Check sheet for the modelled part. Datum: model origin and axes. Units: mm. A direction names the side the tool comes from. Round coordinates to 2 decimals unless told otherwise and drop trailing zeros. Write each loop counter-clockwise with the first axis right and the second up, starting at its lowest first coordinate (ties: lowest second). Pieces come first, ordered by that corner, then holes. Notation, with made-up numbers: (38.5, 39) -> (51.5, 39) arc R23 cw to (51.5, 65) -> close; hole circle Ø11 at (8, -35). An arc over 180 degrees is marked (long way). Answer as a JSON object with one key per item and string values. Group by question number.
```python
from build123d import *

# Parameters (mm, degrees)
SKETCH_1_W      = 12.4
SKETCH_1_H      = 5
SKETCH_1_R      = 1.25
SKETCH_1_W_2    = 5
SKETCH_1_H_2    = 11.3
EXTRUDE_1_DEPTH = 3
SKETCH_2_W      = 3
SKETCH_2_H      = 16.3
EXTRUDE_2_DEPTH = 12
EXTRUDE_3_DEPTH = 2
SKETCH_4_R      = 30
SKETCH_4_R_2    = 1.5
SKETCH_4_R_3    = 6
EXTRUDE_4_DEPTH = 2
FILLET_2_R      = 2


with BuildPart() as part:
    # Эскиз1 → Бобышка-Вытянуть1 (new body)
    with BuildSketch(Plane.XY):
        with Locations((0, 13.8)):
            Rectangle(SKETCH_1_W, SKETCH_1_H)
        with Locations((0, 13.8)):
            Circle(SKETCH_1_R, mode=Mode.SUBTRACT)
        with Locations((8.7, 13.8)):
            Rectangle(SKETCH_1_W_2, SKETCH_1_H)
        with Locations((8.7, 5.65)):
            Rectangle(SKETCH_1_W_2, SKETCH_1_H_2)
    extrude_1 = extrude(amount=EXTRUDE_1_DEPTH)

    # Эскиз2 → Бобышка-Вытянуть2 (add)
    with BuildSketch(Plane(origin=(11.2, 0, 0), x_dir=(0, 0, -1), z_dir=(1, 0, 0))):
        with Locations((-1.5, 8.15)):
            Rectangle(SKETCH_2_W, SKETCH_2_H)
    extrude_2 = extrude(amount=EXTRUDE_2_DEPTH)

    # Эскиз3 → Бобышка-Вытянуть3 (add)
    with BuildSketch(Plane(origin=(0, 16.3, 0), x_dir=(1, 0, 0), z_dir=(0, 1, 0))):
        Polygon((23.2, -8), (23.2, -3), (6.75, -3), align=None)
    extrude_3 = extrude(amount=-EXTRUDE_3_DEPTH)

    # Зеркальное отражение1: Бобышка-Вытянуть1, Бобышка-Вытянуть2, Бобышка-Вытянуть3 across plane
    add(extrude_1.mirror(Plane(origin=(0, 0, 3), x_dir=(0, 0, 1), z_dir=(0, -1, 0))))
    add(extrude_2.mirror(Plane(origin=(0, 0, 3), x_dir=(0, 0, 1), z_dir=(0, -1, 0))))
    add(extrude_3.mirror(Plane(origin=(0, 0, 3), x_dir=(0, 0, 1), z_dir=(0, -1, 0))))

    # Эскиз4 → Бобышка-Вытянуть4 (add)
    with BuildSketch(Plane(origin=(23.2, 0, 0), x_dir=(0, 0, -1), z_dir=(1, 0, 0))):
        with Locations((-23.25, 0)):
            Circle(SKETCH_4_R)
        with Locations((-30, -11.691342951)):
            Circle(SKETCH_4_R_2, mode=Mode.SUBTRACT)
        with Locations((-16.5, 11.691342951)):
            Circle(SKETCH_4_R_2, mode=Mode.SUBTRACT)
        with Locations((-9.75, 0)):
            Circle(SKETCH_4_R_2, mode=Mode.SUBTRACT)
        with Locations((-36.75, 0)):
            Circle(SKETCH_4_R_2, mode=Mode.SUBTRACT)
        with Locations((-16.5, -11.691342951)):
            Circle(SKETCH_4_R_2, mode=Mode.SUBTRACT)
        with Locations((-30, 11.691342951)):
            Circle(SKETCH_4_R_2, mode=Mode.SUBTRACT)
        with Locations((-23.25, 0)):
            Circle(SKETCH_4_R_3, mode=Mode.SUBTRACT)
        Polygon((-3, 14.3), (-3, -14.3), (-8, -14.3), (-8, -16.3), (0, -16.3), (0, 16.3), (-8, 16.3), (-8, 14.3), align=None, mode=Mode.SUBTRACT)
        Polygon((-8, 14.3), (-3, 14.3), (-3, -14.3), (-8, -14.3), (-8, -16.3), (0, -16.3), (0, 16.3), (-8, 16.3), align=None)
    extrude(amount=EXTRUDE_4_DEPTH)

    # Скругление2
    fillet_2_edges = [part.edges().sort_by_distance(p)[0] for p in [
        (23.2, 16.3, 4),
        (23.2, 0, 3),
        (23.2, 15.3, 8),
        (23.2, 14.3, 5.5),
        (23.2, -16.3, 4),
        (23.2, -14.3, 5.5),
        (23.2, -15.3, 8),
    ]]
    fillet(fillet_2_edges, radius=FILLET_2_R)


solid = part.part
```
(1) Section check C-C on z = 23.25. Record the cut outline in (x, y).
(2) Access from +Z, -Z, +X, -X, +Y, -Y to the whole of each face (thin tool, end or side, straight path). Record for faces 4 (the cylindrical face through (24.19, 0.07, 11.25)), 5 (the flat face through (10, 16.3, 2)), 6 (the flat face through (17, 14.3, 4)), 7 (the flat face through (12, -4, 0)), 8 (the flat face through (10, -16.3, 2)).
(3) Scan lines: line 1 along Y through (x, z) = (0, 0.9); line 2 along Y through (x, z) = (24.8, 30); line 3 along Z through (x, y) = (7.5, 11). Record each from-to range of solid material in increasing order.
(4) Section check A-A on x = -3. Record the cut outline in (y, z), then the cut area to 3 significant figures.
(5) Section check B-B on y = 0. Record the cut outline in (x, z), then the cut area to 3 significant figures.
(6) Release check for a two-part mould opening along X. For faces 1 (the flat face through (-6.2, -14, 1)), 2 (the flat face through (17, -14.3, 4)), 3 (the cylindrical face through (-0.27, 12.58, 1.48)) record: pulls with the +X half, pulls with the -X half, needs draft (parallel to the pull), parting line crosses it, or undercut.
(7) Go/stop test with flat-tipped pins: pin 1 Ø6 at (x, z) = (3.5, 4) entering from +Y; pin 2 Ø15.5 at (y, z) = (0, 23.25) entering from -X; pin 3 Ø8 at (x, y) = (4.5, -6) entering from +Z. Record where each tip stops, or that it passes through.
(8) Section check D-D on z = 30. Record the cut outline in (x, y), then the cut area to 3 significant figures.
Data:
{
 "1": {"outline": "(23.2, -30) -> (25.2, -30) -> (25.2, -6) -> (23.2, -6) -> close; (23.2, 6) -> (25.2, 6) -> (25.2, 30) -> (23.2, 30) -> close"},
 "2": {"face 4": "+X, -X", "face 5": "+Z, -Z, -X, +Y", "face 6": "+Z, -X", "face 7": "-Z, -X, +Y, -Y", "face 8": "+Z, -Z, -X, -Y"},
 "3": {"line 1": "y = -16.3 to -15.05, -12.55 to -11.3, 11.3 to 12.55, 15.05 to 16.3", "line 2": "y = -29.23 to -13.19, -10.19 to 10.19, 13.19 to 29.23", "line 3": "z = 0 to 3"},
 "4": {"outline": "(-16.3, 0) -> (-11.3, 0) -> (-11.3, 3) -> (-16.3, 3) -> close; (11.3, 0) -> (16.3, 0) -> (16.3, 3) -> (11.3, 3) -> close", "area": "30.0 mm²"},
 "5": {"outline": "(6.2, 0) -> (23.2, 0) -> (23.2, -6.75) -> (25.2, -6.75) -> (25.2, 8.25) -> (23.2, 8.25) -> (23.2, 5) arc R2 cw to (21.2, 3) -> (6.2, 3) -> close; (23.2, 11.25) -> (25.2, 11.25) -> (25.2, 17.25) -> (23.2, 17.25) -> close; (23.2, 29.25) -> (25.2, 29.25) -> (25.2, 35.25) -> (23.2, 35.25) -> close; (23.2, 38.25) -> (25.2, 38.25) -> (25.2, 53.25) -> (23.2, 53.25) -> close", "area": "136 mm²"},
 "6": {"face 1": "pulls with the -X half", "face 2": "needs draft", "face 3": "undercut"},
 "7": {"pin 1": "stops at y = 16.3", "pin 2": "stops at x = 23.2", "pin 3": "stops at z = 3"},
 "8": {"outline": "(23.2, -29.23) -> (25.2, -29.23) -> (25.2, -13.19) -> (23.2, -13.19) -> close; (23.2, -10.19) -> (25.2, -10.19) -> (25.2, 10.19) -> (23.2, 10.19) -> close; (23.2, 13.19) -> (25.2, 13.19) -> (25.2, 29.23) -> (23.2, 29.23) -> close", "area": "105 mm²"}
}
